from build123d import *

# Parameters (mm, degrees)
SKETCH4_R          = 10
CUT_EXTRUDE1_DEPTH = 22


# Read off the part's stored shape, not the designer's step: Shell4
with BuildPart() as part:
    # Sketch2 → Revolve3 (revolve)
    with BuildSketch(Plane.XY):
        with BuildLine():
            ThreePointArc((-75, 0), (-38.854521396, 15.079455235), (0, 20))
            Line((0, 20), (0, 0))
            Line((0, 0), (-75, 0))
        make_face()
    revolve(axis=Axis((0, 20, 0), (0, -1, 0)))

    # Shell4 outline → Shell4 (revolve, cut)
    with BuildSketch(Plane.XY):
        with BuildLine():
            Line((0, 0), (70.959299581, 0))
            add(Edge.make_bspline(
                [(70.959299581, 0), (58.371091625, 6.969352493), (44.697655968, 12.48291706), (30.310219449, 16.202186231), (15.668630532, 18.005474405), (1.010939764, 18.005474483), (0.758094755, 18.004918806), (0.505321529, 18.00380806), (0.252622481, 18.002142877), (0, 17.999923905)],
                knots=[1.06516175, 1.06516175, 1.06516175, 1.06516175, 1.06516175, 1.06516175, 1.570703705, 1.570703705, 1.570703705, 1.570703705, 1.579579846, 1.579579846, 1.579579846, 1.579579846, 1.579579846, 1.579579846], degree=5, weights=[1, 1, 0.999596269, 0.999595367, 1, 1, 1, 1, 1, 1]))
            Line((0, 17.999923905), (0, 0))
        make_face()
    revolve(axis=Axis((0, 0, 0), (0, 1, 0)), mode=Mode.SUBTRACT)

    # Sketch4 → Cut-Extrude1 (cut)
    with BuildSketch(Plane(origin=(0, 0, 0), x_dir=(1, 0, 0), z_dir=(0, 1, 0))):
        with Locations(Location((0, 0, 0), (0, 0, 90))):
            Circle(SKETCH4_R)
    extrude(amount=CUT_EXTRUDE1_DEPTH, mode=Mode.SUBTRACT)


solid = part.part
Work out the finished part from the listing and answer in its coordinate system (mm). Give positions to 0.01 mm unless a question says otherwise; leave off trailing zeros. One line per item, written item: value. Start each with the question number.
1. Consider probe 1 along Z at (x, y) = (-17, 2); probe 2 along X at (y, z) = (1, -31); probe 3 along Z at (x, y) = (-6.5, 2.75). Determine where each line is inside the solid, lowest interval first.
2. Given pin 1 (10 mm diameter, centred on x = -17.5, z = -2.5, fed in from +Y); pin 2 (2 mm diameter, centred on x = 42.5, z = -56, fed in from -Y); pin 3 (2 mm diameter, centred on x = -13, z = 52.5, fed in from -Y); pin 4 (12 mm diameter, centred on x = 56.5, z = 26.5, fed in from +Y), each flat-ended and moving along its own axis, determine where each tip first touches the part or whether it passes through.
3. For a pull along X with two mould halves and no side action, classify faces 1 (the cylindrical face through (9.76, 18.73, 2.17)), 2 (the flat face through (66, 0, 27)) as +X half, -X half, draft (parallel to the pull), parting line (faces both ways), or undercut.
Geometry results:
1. probe 1: -69.42 to -65.03, 65.03 to 69.42
1. probe 2: -66.38 to -61.78, 61.78 to 66.38
1. probe 3: -69.79 to -65.42, 65.42 to 69.79
2. pin 1: y = 19.56
2. pin 2: y = 0
2. pin 3: y = 7.56
2. pin 4: y = 9.18
3. face 1: undercut
3. face 2: draft
